The model under review builds one solid part; all positions refer to its coordinate system, in mm. A direction names the side the tool comes from. Coordinates: 2 decimals unless noted, no trailing zeros. Write each loop counter-clockwise with the first axis right and the second up, starting at its lowest first coordinate (ties: lowest second). Pieces come first, ordered by that corner, then holes. Notation, with made-up numbers: (20.5, 22.5) - (31.5, 22.5) arc R22 ccw to (31.5, 36.5) - close; hole circle Ø2 at (36.25, 54.5). An arc over 180 degrees is marked (long way). Put each result on its own line as item: value. Start each with the question number.
Item 1: Consider section D-D on z = -0.5. Give the boundary of the cut face in (x, y), then the cut area to 3 significant figures.
Item 2: Consider section A-A on z = 58. Give the boundary of the cut face in (x, y).
Item 3: Consider section C-C on y = 1.8. State how many separate pieces and enclosed holes the cut face has, then the cut area to 3 significant figures.
Item 4: To check wall thickness, follow L1, parallel to X at y = 0.1, z = 42; L2, parallel to X at y = 1.05, z = -15; L3, parallel to X at y = 1.5, z = -41. State the ranges of each line that lie inside material, in increasing order. Write a range as [from, to].
Item 5: Machinability: for faces 3 (the face through (-4.056, 1.479, 21.408)), 4 (the face through (47.921, 1.479, -39.436)), 5 (the face through (-21.565, 1.479, 12.4)), which of the approach directions +Z, -Z, +X, -X, +Y, -Y give a long, thin tool a straight path to every point of the face, cutting with its end or side? Answer none if there is none.
Item 6: Consider section B-B on x = 56.5. Give the boundary of the cut face in (y, z), then the cut area to 3 significant figures.
Item 7: Mouldability with a two-part tool opening along Z and no side actions: class faces 1 (the face through (4.06, 1.48, 18.52)), 2 (the face through (-81.908, 1.479, -93.712)) as pulls with the +Z half, pulls with the -Z half, needs draft (parallel to the pull), parting line crosses it, or undercut.
Item 8: For pin 1 (0.9 mm diameter, centred on y = 2, z = 2.5, fed in from +X); pin 2 (2 mm diameter, centred on x = -1, z = 7, fed in from -Y); pin 3 (1.5 mm diameter, centred on x = 68, y = 1, fed in from +Z); pin 4 (0.9 mm diameter, centred on y = 1.5, z = -22.5, fed in from -X), all flat-tipped, find the tip position at first contact; note any pin that passes through.
```python
from build123d import *

# Parameters (mm, degrees)
SKETCH1_R           = 1.6
SKETCH1_R_2         = 5
BOSS_EXTRUDE1_DEPTH = 3
CUT_EXTRUDE1_DEPTH  = 137.389779764


with BuildPart() as part:
    # Sketch1 → Boss-Extrude1 (new body)
    with BuildSketch(Plane(origin=(0, 0, 0), x_dir=(1, 0, 0), z_dir=(0, 1, 0))):
        with BuildLine():
            Line((19.341013177, -38.656931626), (16.02192173, -47.77606043))
            ThreePointArc((16.02192173, -47.77606043), (14.923573177, -49.207456133), (13.202843868, -49.75))
            Line((13.202843868, -49.75), (-13.202843868, -49.75))
            ThreePointArc((-13.202843868, -49.75), (-14.923573177, -49.207456133), (-16.02192173, -47.77606043))
            Line((-16.02192173, -47.77606043), (-19.944086969, -37))
            Line((-19.944086969, -37), (-19.944086969, -34.257795468))
            ThreePointArc((-19.944086969, -34.257795468), (-21.796036672, -31.486156871), (-25.065407313, -32.136475125))
            Line((-25.065407313, -32.136475125), (-60.998570725, -68.069638537))
            ThreePointArc((-60.998570725, -68.069638537), (-63.363139484, -71.828794135), (-63.866770837, -76.241139508))
            ThreePointArc((-63.866770837, -76.241139508), (-66.073761636, -85.457884527), (-73.646067483, -91.156952986))
            Line((-73.646067483, -91.156952986), (-89.941777265, -96.195664945))
            ThreePointArc((-89.941777265, -96.195664945), (-94.954339188, -94.954339188), (-96.195664945, -89.941777265))
            Line((-96.195664945, -89.941777265), (-91.156952986, -73.646067483))
            ThreePointArc((-91.156952986, -73.646067483), (-85.457884527, -66.073761636), (-76.241139508, -63.866770837))
            ThreePointArc((-76.241139508, -63.866770837), (-71.828794135, -63.363139484), (-68.069638537, -60.998570725))
            Line((-68.069638537, -60.998570725), (-25.857864376, -18.786796564))
            ThreePointArc((-25.857864376, -18.786796564), (-21.52240935, -12.298329588), (-20, -4.644660941))
            Line((-20, -4.644660941), (-20, 3.230447378))
            ThreePointArc((-20, 3.230447378), (-21.52240935, 10.884116026), (-25.857864376, 17.372583002))
            Line((-25.857864376, 17.372583002), (-69.375275977, 60.889994603))
            ThreePointArc((-69.375275977, 60.889994603), (-72.878122891, 63.16065038), (-77.002761348, 63.803434766))
            ThreePointArc((-77.002761348, 63.803434766), (-85.774590221, 66.287641348), (-91.156952986, 73.646067483))
            Line((-91.156952986, 73.646067483), (-96.195664945, 89.941777265))
            ThreePointArc((-96.195664945, 89.941777265), (-94.954339188, 94.954339188), (-89.941777265, 96.195664945))
            Line((-89.941777265, 96.195664945), (-73.646067483, 91.156952986))
            ThreePointArc((-73.646067483, 91.156952986), (-66.287641348, 85.774590221), (-63.803434766, 77.002761348))
            ThreePointArc((-63.803434766, 77.002761348), (-63.16065038, 72.878122891), (-60.889994603, 69.375275977))
            Line((-60.889994603, 69.375275977), (-25.121320344, 33.606601718))
            ThreePointArc((-25.121320344, 33.606601718), (-21.851949703, 32.956283464), (-20, 35.727922061))
            Line((-20, 35.727922061), (-20, 37))
            ThreePointArc((-20, 37), (-18.535533906, 40.535533906), (-15, 42))
            Line((-15, 42), (15, 42))
            ThreePointArc((15, 42), (18.535533906, 40.535533906), (20, 37))
            Line((20, 37), (20, 35.727922061))
            ThreePointArc((20, 35.727922061), (21.851949703, 32.956283464), (25.121320344, 33.606601718))
            Line((25.121320344, 33.606601718), (60.889994603, 69.375275977))
            ThreePointArc((60.889994603, 69.375275977), (63.16065038, 72.878122891), (63.803434766, 77.002761348))
            ThreePointArc((63.803434766, 77.002761348), (66.287641348, 85.774590221), (73.646067483, 91.156952986))
            Line((73.646067483, 91.156952986), (89.941777265, 96.195664945))
            ThreePointArc((89.941777265, 96.195664945), (94.954339188, 94.954339188), (96.195664945, 89.941777265))
            Line((96.195664945, 89.941777265), (91.156952986, 73.646067483))
            ThreePointArc((91.156952986, 73.646067483), (85.774590221, 66.287641348), (77.002761348, 63.803434766))
            ThreePointArc((77.002761348, 63.803434766), (72.878122891, 63.16065038), (69.375275977, 60.889994603))
            Line((69.375275977, 60.889994603), (25.857864376, 17.372583002))
            ThreePointArc((25.857864376, 17.372583002), (21.52240935, 10.884116026), (20, 3.230447378))
            Line((20, 3.230447378), (20, -4.644660941))
            ThreePointArc((20, -4.644660941), (21.52240935, -12.298329588), (25.857864376, -18.786796564))
            Line((25.857864376, -18.786796564), (68.069638537, -60.998570725))
            ThreePointArc((68.069638537, -60.998570725), (71.828794135, -63.363139484), (76.241139508, -63.866770837))
            ThreePointArc((76.241139508, -63.866770837), (85.457884527, -66.073761636), (91.156952986, -73.646067483))
            Line((91.156952986, -73.646067483), (96.195664945, -89.941777265))
            ThreePointArc((96.195664945, -89.941777265), (94.954339188, -94.954339188), (89.941777265, -96.195664945))
            Line((89.941777265, -96.195664945), (73.646067483, -91.156952986))
            ThreePointArc((73.646067483, -91.156952986), (66.073761636, -85.457884527), (63.866770837, -76.241139508))
            ThreePointArc((63.866770837, -76.241139508), (63.363139484, -71.828794135), (60.998570725, -68.069638537))
            Line((60.998570725, -68.069638537), (25.065407313, -32.136475125))
            ThreePointArc((25.065407313, -32.136475125), (21.796036672, -31.486156871), (19.944086969, -34.257795468))
            Line((19.944086969, -34.257795468), (19.944086969, -35.236730193))
            ThreePointArc((19.944086969, -35.236730193), (19.792164499, -36.97321197), (19.341013177, -38.656931626))
        make_face()
        with Locations(Location((77.781745931, 68.281745931, 0), (0, 0, 270))):
            Circle(SKETCH1_R, mode=Mode.SUBTRACT)
        with Locations(Location((68.281745931, 77.781745931, 0), (0, 0, 270))):
            Circle(SKETCH1_R, mode=Mode.SUBTRACT)
        with Locations(Location((77.781745931, 87.281745931, 0), (0, 0, 270))):
            Circle(SKETCH1_R, mode=Mode.SUBTRACT)
        with Locations(Location((87.281745931, 77.781745931, 0), (0, 0, 270))):
            Circle(SKETCH1_R, mode=Mode.SUBTRACT)
        with Locations(Location((77.781745931, -87.281745931, 0), (0, 0, 270))):
            Circle(SKETCH1_R, mode=Mode.SUBTRACT)
        with Locations(Location((68.281745931, -77.781745931, 0), (0, 0, 270))):
            Circle(SKETCH1_R, mode=Mode.SUBTRACT)
        with Locations(Location((77.781745931, -68.281745931, 0), (0, 0, 270))):
            Circle(SKETCH1_R, mode=Mode.SUBTRACT)
        with Locations(Location((87.281745931, -77.781745931, 0), (0, 0, 270))):
            Circle(SKETCH1_R, mode=Mode.SUBTRACT)
        with Locations(Location((15, 15, 0), (0, 0, 270))):
            Circle(SKETCH1_R, mode=Mode.SUBTRACT)
        with Locations(Location((15, -15, 0), (0, 0, 270))):
            Circle(SKETCH1_R, mode=Mode.SUBTRACT)
        with Locations(Location((77.781745931, 77.781745931, 0), (0, 0, 270))):
            Circle(SKETCH1_R_2, mode=Mode.SUBTRACT)
        with Locations(Location((77.781745931, -77.781745931, 0), (0, 0, 270))):
            Circle(SKETCH1_R_2, mode=Mode.SUBTRACT)
        with Locations(Location((14.944086969, -37, 0), (0, 0, 90))):
            Circle(SKETCH1_R, mode=Mode.SUBTRACT)
        with Locations(Location((15, 37, 0), (0, 0, 90))):
            Circle(SKETCH1_R, mode=Mode.SUBTRACT)
        with Locations(Location((-15, 37, 0), (0, 0, 270))):
            Circle(SKETCH1_R, mode=Mode.SUBTRACT)
        with Locations(Location((-14.944086969, -37, 0), (0, 0, 270))):
            Circle(SKETCH1_R, mode=Mode.SUBTRACT)
        with Locations(Location((-77.781745931, -77.781745931, 0), (0, 0, 90))):
            Circle(SKETCH1_R_2, mode=Mode.SUBTRACT)
        with Locations(Location((-77.781745931, 77.781745931, 0), (0, 0, 90))):
            Circle(SKETCH1_R_2, mode=Mode.SUBTRACT)
        with Locations(Location((-15, -15, 0), (0, 0, 90))):
            Circle(SKETCH1_R, mode=Mode.SUBTRACT)
        with Locations(Location((-15, 15, 0), (0, 0, 90))):
            Circle(SKETCH1_R, mode=Mode.SUBTRACT)
        with Locations(Location((-87.281745931, -77.781745931, 0), (0, 0, 90))):
            Circle(SKETCH1_R, mode=Mode.SUBTRACT)
        with Locations(Location((-77.781745931, -68.281745931, 0), (0, 0, 90))):
            Circle(SKETCH1_R, mode=Mode.SUBTRACT)
        with Locations(Location((-68.281745931, -77.781745931, 0), (0, 0, 90))):
            Circle(SKETCH1_R, mode=Mode.SUBTRACT)
        with Locations(Location((-77.781745931, -87.281745931, 0), (0, 0, 90))):
            Circle(SKETCH1_R, mode=Mode.SUBTRACT)
        with Locations(Location((-87.281745931, 77.781745931, 0), (0, 0, 90))):
            Circle(SKETCH1_R, mode=Mode.SUBTRACT)
        with Locations(Location((-77.781745931, 87.281745931, 0), (0, 0, 90))):
            Circle(SKETCH1_R, mode=Mode.SUBTRACT)
        with Locations(Location((-68.281745931, 77.781745931, 0), (0, 0, 90))):
            Circle(SKETCH1_R, mode=Mode.SUBTRACT)
        with Locations(Location((-77.781745931, 68.281745931, 0), (0, 0, 90))):
            Circle(SKETCH1_R, mode=Mode.SUBTRACT)
    extrude(amount=BOSS_EXTRUDE1_DEPTH)

    # Sketch2 → Cut-Extrude1 (cut, through all)
    with BuildSketch(Plane.XZ):
        Polygon((-8, 35.131197846), (0, 39.75), (8, 35.131197846), (8, 32.244446501), (0, 36.863248654), (-8, 32.244446501), align=None)
        Polygon((-8, 27.131197846), (0, 31.75), (8, 27.131197846), (8, 24.244446501), (0, 28.863248654), (-8, 24.244446501), align=None)
        Polygon((-8, 19.131197846), (0, 23.75), (8, 19.131197846), (8, 16.244446501), (0, 20.863248654), (-8, 16.244446501), align=None)
        Polygon((-8, -12.868802154), (0, -8.25), (8, -12.868802154), (8, -15.755553499), (0, -11.136751346), (-8, -15.755553499), align=None)
        Polygon((-8, -20.868802154), (0, -16.25), (8, -20.868802154), (8, -23.755553499), (0, -19.136751346), (-8, -23.755553499), align=None)
        Polygon((-8, -28.868802154), (0, -24.25), (8, -28.868802154), (8, -31.755553499), (0, -27.136751346), (-8, -31.755553499), align=None)
    extrude(amount=-CUT_EXTRUDE1_DEPTH, mode=Mode.SUBTRACT)


solid = part.part
```
Report:
1. outline: (-20, 0) - (20, 0) - (20, 3) - (-20, 3) - close
1. area: 120 mm²
2. outline: (-65.07, 0) - (-50.93, 0) - (-50.93, 3) - (-65.07, 3) - close; (50.93, 0) - (65.07, 0) - (65.07, 3) - (50.93, 3) - close
3. separate pieces: 1
3. enclosed holes: 34
3. area: 8,940 mm²
4. L1: [-49.07, -34.93], [-18.12, 18.12], [34.93, 49.07]
4. L2: [-23.83, -16.6], [-13.4, -8], [-6.69, 6.69], [8, 13.4], [16.6, 23.83]
4. L3: [-49.49, -32.51], [-18, 18], [32.51, 49.49]
5. face 3: +Y, -Y
5. face 4: +X, +Y, -Y
5. face 5: -X, +Y, -Y
6. outline: (0, -64.99) - (3, -64.99) - (3, -48.01) - (0, -48.01) - close; (0, 49.43) - (3, 49.43) - (3, 63.57) - (0, 63.57) - close
6. area: 93.3 mm²
7. face 1: undercut
7. face 2: pulls with the -Z half
8. pin 1: x = 20
8. pin 2: y = 0
8. pin 3: z = 88.48
8. pin 4: x = -31.44
